Geometry check sheet. Reference: the model listing, model coordinates, mm. Round coordinates to 2 decimals unless told otherwise and drop trailing zeros. Write each loop counter-clockwise with the first axis right and the second up, starting at its lowest first coordinate (ties: lowest second). Pieces come first, ordered by that corner, then holes. Notation, with made-up numbers: (42.25, 73.25) -> (55.25, 73.25) arc R19 cw to (55.25, 102.25) -> close; hole circle Ø7 at (3, -3). An arc over 180 degrees is marked (long way). One line per question, with ' | ' between items.
```python
from build123d import *

# Parameters (mm, degrees)
F0_R     = 2
F1_DEPTH = 5
F2_SIZE2 = 39.99999
F2_SIZE  = 4.99999


# Not quite as in the source:
# - a fillet or chamfer is up to 0.001 mm smaller than in the source, because OpenCascade refuses the exact size


with BuildPart() as f1:
    # F0 (on Top) → F1 (new body)
    with BuildSketch(Plane.XY):
        with BuildLine():
            Line((1, 72.995454073), (0, 72.995454073))
            Line((0, 72.995454073), (-1, 72.995454073))
            Line((-1, 72.995454073), (-6.690328202, 13.4253308544))
            ThreePointArc((-6.690328202, 13.4253308544), (0, 15), (6.690328202, 13.4253308544))
            Line((6.690328202, 13.4253308544), (1, 72.995454073))
        make_face()
        with BuildLine():
            ThreePointArc((15, 0), (12.7545074979, 7.8944625204), (6.690328202, 13.4253308544))
            Line((6.690328202, 13.4253308544), (2.3585444492, -14.813415139))
            ThreePointArc((2.3585444492, -14.813415139), (11.4100430923, -9.7370897413), (15, 0))
        make_face()
        with BuildLine():
            Line((2.3585444492, -14.813415139), (6.690328202, 13.4253308544))
            ThreePointArc((6.690328202, 13.4253308544), (0, 15), (-6.690328202, 13.4253308544))
            Line((-6.690328202, 13.4253308544), (-2.3585444492, -14.813415139))
            ThreePointArc((-2.3585444492, -14.813415139), (0, -15), (2.3585444492, -14.813415139))
        make_face()
        Circle(F0_R, mode=Mode.SUBTRACT)
        with BuildLine():
            Line((-2.3585444492, -14.813415139), (-6.690328202, 13.4253308544))
            ThreePointArc((-6.690328202, 13.4253308544), (-14.8265713462, -2.2743751044), (-2.3585444492, -14.813415139))
        make_face()
        with BuildLine():
            Line((2, -59.9238947034), (2.3585444492, -14.813415139))
            ThreePointArc((2.3585444492, -14.813415139), (0, -15), (-2.3585444492, -14.813415139))
            Line((-2.3585444492, -14.813415139), (-2, -59.9238947034))
            Line((-2, -59.9238947034), (0, -59.9238947034))
            Line((0, -59.9238947034), (2, -59.9238947034))
        make_face()
    extrude(amount=F1_DEPTH)

    # F2 (size 5 and 40 in the source; OpenCascade refuses exactly that, so slightly less here)
    f2_edges = [f1.edges().sort_by_distance(p)[0] for p in [
        (0, 72.995454, 5),
    ]]
    f2_side = f1.faces().sort_by_distance((0, 72.995454, 2.5))[0]
    chamfer(f2_edges, length=F2_SIZE, length2=F2_SIZE2, reference=f2_side)


solid = f1.part
```
(1) Material ranges on line 1 (Z direction, x = -1.5, y = 50.5); line 2 (X direction, y = -47, z = 2.2); line 3 (X direction, y = 5, z = 2.65), recorded low to high.
Resolved:
line 1: z = 0 to 2.81 | line 2: x = -2.1 to 2.1 | line 3: x = -14.14 to 14.14
(2) Sectioned sample at A-A on z = 2.2. Record the cut outline in (x, y), then the cut area to 3 significant figures.
Resolved:
outline: (-6.69, 13.43) arc R15 ccw to (-2.36, -14.81) -> (-2, -59.92) -> (2, -59.92) -> (2.36, -14.81) arc R15 ccw to (6.69, 13.43) -> (2.68, 55.4) -> (-2.68, 55.4) -> close; hole circle Ø4 at (0, 0) | area: 1,270 mm2
(3) Go/stop test with flat-tipped pins: pin 1 (1 mm diameter, centred on y = -36.5, z = 0.5, fed in from +X); pin 2 (3 mm diameter, centred on y = -36.5, z = 1.5, fed in from -X). Record where each tip stops, or that it passes through.
Resolved:
pin 1: stops at x = 2.19 | pin 2: stops at x = -2.2
(4) Draft check along X on faces 1 (the cylindrical face through (0, -2, 2)), 2 (the flat face through (-0.2, -2.5, 5)), 3 (the flat face through (-4.438, 37.008, 1.909)). Enter one of: +X half, -X half, draft (parallel to the pull), parting line (faces both ways), or undercut.
Resolved:
face 1: undercut | face 2: draft | face 3: -X half
(5) Sectioned sample at C-C on y = -10.5. Record the cut outline in (x, z), then the cut area to 3 significant figures.
Resolved:
outline: (-10.71, 0) -> (10.71, 0) -> (10.71, 5) -> (-10.71, 5) -> close | area: 107 mm2
(6) Sectioned sample at B-B on x = -9. Record the cut outline in (y, z), then the cut area to 3 significant figures.
Resolved:
outline: (-12, 0) -> (12, 0) -> (12, 5) -> (-12, 5) -> close | area: 120 mm2
